Can you work these out from the model? Positions are in its coordinate system, mm. Face numbers are marked on the shaded views. A direction names the side the tool comes from. Give positions to 0.01 mm unless a question says otherwise; leave off trailing zeros. Write each loop counter-clockwise with the first axis right and the second up, starting at its lowest first coordinate (ties: lowest second). Pieces come first, ordered by that corner, then holes. Notation, with made-up numbers: M 78,59.5 L 104,59.5 A23 cw 104,70.5 Z; hole C -14.5,-40 d2. An arc over 180 degrees is marked long. Answer as CSV lines item,"result". Start each with the question number.
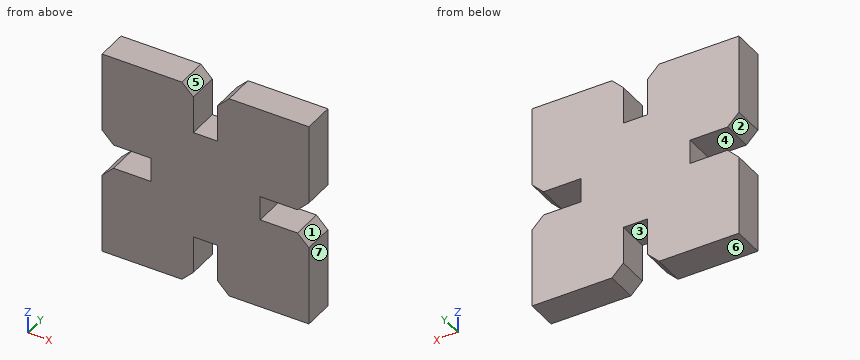
Autodesk Fusion 360 part; units mm, degrees
sketch "Sketch1" plane through (0, 0, 0) normal (0, 1, 0) x (1, 0, 0)
  line L0 (13.6189, 1.605) -> (13.6189, 13.6189)
  line L1 (-13.6189, 13.6189) -> (-13.6189, 1.605)
  line L2 (13.6189, -1.605) -> (13.6189, -13.6189)
  line L3 (-13.6189, -13.6189) -> (-13.6189, -1.605)
  line L4 (1.605, 7.1989) -> (1.605, 13.6189)
  line L5 (0, 0) -> (2.5, 0)
  line L6 (7.1989, 1.605) -> (13.6189, 1.605)
  line L7 (7.1989, -1.605) -> (13.6189, -1.605)
  line L8 (13.6189, 13.6189) -> (1.605, 13.6189)
  line L9 (-1.605, 13.6189) -> (-13.6189, 13.6189)
  line L10 (-13.6189, 13.6189) -> (0, 0)
  line L11 (0, 0) -> (13.6189, 13.6189)
  line L12 (-13.6189, -13.6189) -> (0, 0)
  line L13 (0, 0) -> (13.6189, -13.6189)
  line L14 (7.1989, 1.605) -> (7.1989, -1.605)
  line L15 (-7.1989, -1.605) -> (-13.6189, -1.605)
  line L16 (-7.1989, 1.605) -> (-7.1989, -1.605)
  line L17 (-7.1989, 1.605) -> (-13.6189, 1.605)
  line L18 (-1.605, 7.1989) -> (-1.605, 13.6189)
  line L19 (1.605, 7.1989) -> (-1.605, 7.1989)
  line L20 (-1.605, -7.1989) -> (-1.605, -13.6189)
  line L21 (1.605, -7.1989) -> (1.605, -13.6189)
  line L22 (1.605, -7.1989) -> (-1.605, -7.1989)
  line L23 (13.6189, -13.6189) -> (1.605, -13.6189)
  line L24 (-1.605, -13.6189) -> (-13.6189, -13.6189)
  line L25 (81.6508, 319732.5239) -> (6.33, 319732.5239)
  line L26 (81.6508, 319732.5239) -> (102.864, 319753.7371)
  line L27 (92.864, 319735.0239) -> (102.864, 319735.0239)
  line L28 (102.864, 319753.7371) -> (84.1508, 319753.7371)
  line L29 (92.864, 319730.0239) -> (102.864, 319730.0239)
  line L30 (102.864, 319735.0239) -> (102.864, 319753.7371)
  line L31 (60.4376, 319753.7371) -> (60.4376, 319735.0239)
  line L32 (60.4376, 319711.3107) -> (60.4376, 319730.0239)
  line L33 (84.1508, 319743.7371) -> (84.1508, 319753.7371)
  line L34 (60.4376, 319711.3107) -> (81.6508, 319732.5239)
  line L35 (102.864, 319730.0239) -> (102.864, 319711.3107)
  line L36 (60.4376, 319753.7371) -> (81.6508, 319732.5239)
  line L37 (84.1508, 319721.3107) -> (79.1508, 319721.3107)
  line L38 (84.1508, 319721.3107) -> (84.1508, 319711.3107)
  line L39 (79.1508, 319721.3107) -> (79.1508, 319711.3107)
  line L40 (84.1508, 319743.7371) -> (79.1508, 319743.7371)
  line L41 (79.1508, 319743.7371) -> (79.1508, 319753.7371)
  line L42 (92.864, 319735.0239) -> (92.864, 319730.0239)
  line L43 (81.6508, 319732.5239) -> (102.864, 319711.3107)
  line L44 (79.1508, 319753.7371) -> (60.4376, 319753.7371)
  line L45 (79.1508, 319711.3107) -> (60.4376, 319711.3107)
  line L46 (70.4376, 319730.0239) -> (60.4376, 319730.0239)
  line L47 (70.4376, 319735.0239) -> (70.4376, 319730.0239)
  line L48 (70.4376, 319735.0239) -> (60.4376, 319735.0239)
  line L49 (102.864, 319711.3107) -> (84.1508, 319711.3107)
  dimension "d9" = 19.26
  dimension "d15" = 6.42
  dimension "d60" = 30
  dimension "d61" = 10
  dimension "d62" = 5
  dimension "d69" = 3.21
extrude "Extrude1" add sketch "Sketch1" along normal blind 4.1 contours L0 L2 L6 L7 L11 L13 L14 | L4 L8 L9 L10 L11 L18 L19 | L1 L3 L10 L12 L15 L16 L17 | L12 L13 L20 L21 L22 L23 L24
chamfer "Chamfer1" distance 1.5 angle 45 8 edges at (-13.6189, 2.05, 1.605) (-13.6189, 2.05, -1.605) (-1.605, 2.05, -13.6189) (1.605, 2.05, -13.6189) (13.6189, 2.05, -1.605) (13.6189, 2.05, 1.605) (1.605, 2.05, 13.6189) (-1.605, 2.05, 13.6189) measured on face at (-9.3389, 1.3667, 1.605) measured on face at (-13.6189, 1.3667, -9.6143) measured on face at (-1.605, 2.7333, -11.4789) measured on face at (9.6143, 1.3667, -13.6189) measured on face at (9.3389, 1.3667, -1.605) measured on face at (13.6189, 1.3667, 5.6096) measured on face at (1.605, 1.3667, 9.3389) measured on face at (-5.6096, 1.3667, 13.6189)
equation "d9 = THICKNESS * 6"
equation "d15 = THICKNESS * 2"
equation "SLOT = 10 mm"
equation "d60 = SLOT * 3"
equation "d61 = SLOT"
equation "d62 = SLOT / 2"
equation "d69 = THICKNESS"
equation "THICKNESS = 3.21 mm"
1) I want a section at B-B, the plane x = 8.25. Please give me the cut outline in (y, z) (3 decimals).
2) I want a section at D-D, the plane x = 0.25. Please give me the cut outline in (y, z).
3) On a 3-axis mill with a long thin cutter (end or side, diameter ignored), from which of +Z, -Z, +X, -X, +Y, -Y can I reach the whole of each face in a straight line? I mean the marked faces 1, 2 and 3. Say none if no direction works.
4) I'm going to push flat-ended pins straight in: P1, Ø1.6, axis at x = 0.5, y = 2.5, coming from the +Z side; P2, Ø1.6, axis at y = 3, z = 0.5, coming from the -X side; P3, Ø1, axis at y = 2, z = 1.5, coming from the +X side. Where does each tip first touch, or does it pass through?
5) I want a section at C-C, the plane y = 3.3. Please give me the cut outline in (x, z) (3 decimals).
6) I want a section at A-A, the plane z = -10. Please give me the cut outline in (x, y) (3 decimals), then the cut area to 3 significant figures.
7) Thinking about a two-plate mould opening in Z: for the marked faces 4, 5, 6 and 7, which applies, released by +Z, released by -Z, zero draft, split by the parting line, or undercut?
8) I need wall thicknesses on L1, parallel to Z at x = -8, y = 2.75 (3 decimals); L2, parallel to X at y = 3.45, z = -0.75. Which ranges of each line are inside material? Lowest first, please. Write a range as from..to.
Values found:
1,outline,"M 0,-13.619 L 4.1,-13.619 L 4.1,-1.605 L 0,-1.605 Z; M 0,1.605 L 4.1,1.605 L 4.1,13.619 L 0,13.619 Z"
2,outline,"M 0,-7.2 L 4.1,-7.2 L 4.1,7.2 L 0,7.2 Z"
3,face 1,"+X, +Y, -Y"
3,face 2,"-X, +Y, -Y"
3,face 3,"-Z, +Y, -Y"
4,P1,"stops at z = 7.2"
4,P2,"stops at x = -7.2"
4,P3,"stops at x = 12.51"
5,outline,"M -13.619,-13.619 L -3.105,-13.619 L -1.605,-12.119 L -1.605,-7.199 L 1.605,-7.199 L 1.605,-12.119 L 3.105,-13.619 L 13.619,-13.619 L 13.619,-3.105 L 12.119,-1.605 L 7.199,-1.605 L 7.199,1.605 L 12.119,1.605 L 13.619,3.105 L 13.619,13.619 L 3.105,13.619 L 1.605,12.119 L 1.605,7.199 L -1.605,7.199 L -1.605,12.119 L -3.105,13.619 L -13.619,13.619 L -13.619,3.105 L -12.119,1.605 L -7.199,1.605 L -7.199,-1.605 L -12.119,-1.605 L -13.619,-3.105 Z"
6,outline,"M -13.619,0 L -1.605,0 L -1.605,4.1 L -13.619,4.1 Z; M 1.605,0 L 13.619,0 L 13.619,4.1 L 1.605,4.1 Z"
6,area,"98.5 mm²"
7,face 4,"undercut"
7,face 5,"released by +Z"
7,face 6,"released by -Z"
7,face 7,"zero draft"
8,L1,"z = -13.619..-1.605, 1.605..13.619"
8,L2,"x = -7.2..7.2"
